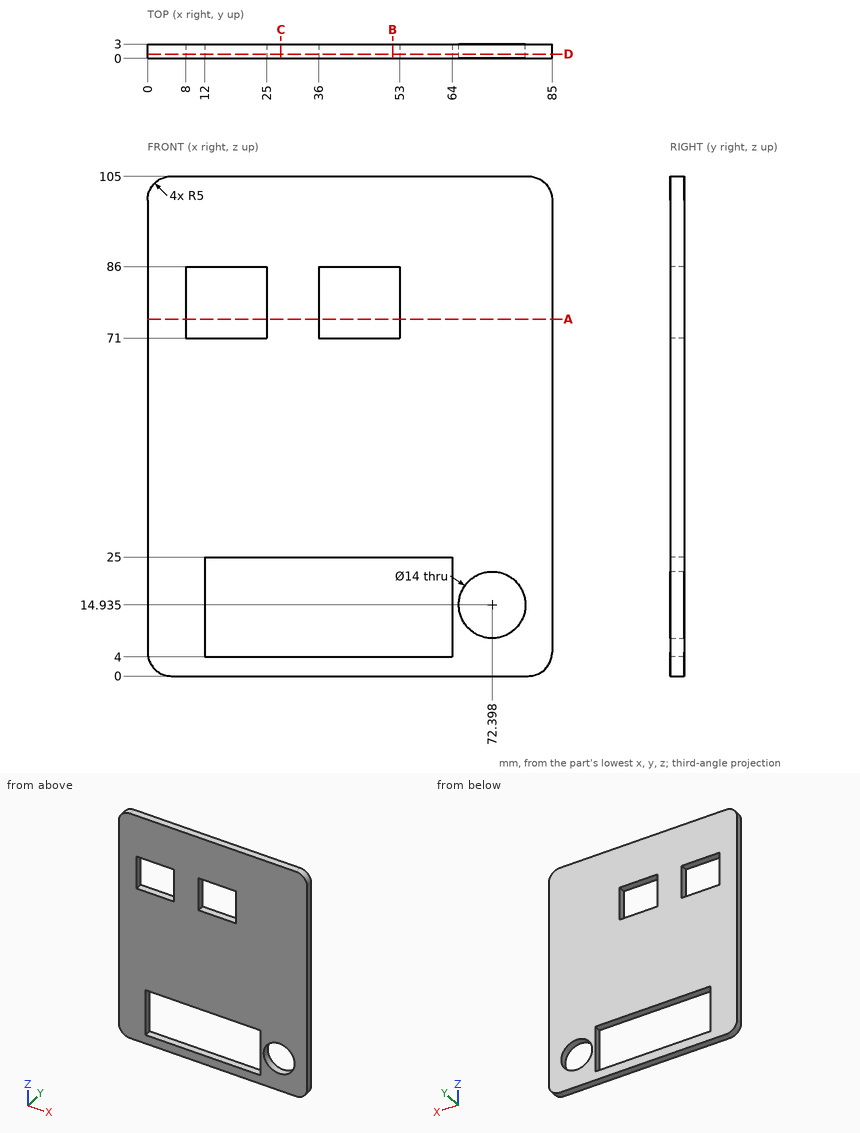
For this review, use the dimensioned drawing (mm, ordinates from the lowest corner) and the shaded views. Give positions to 0.01 mm unless a question says otherwise; leave off trailing zeros. Order: outer loops, then holes, each group sorted by start corner. A loop starts at its lowest first (then second) coordinate and runs counter-clockwise, first axis right, second up.
1) Take a section at A-A (z = 75). Give the boundary of the cut face in (x, y).
2) Take a section at B-B (x = 51.5). Give the boundary of the cut face in (y, z).
3) Wall thickness on line 1 (Z direction, x = 50.5, y = 1.4); line 2 (X direction, y = 2.05, z = 74.5); line 3 (Z direction, x = 54.5, y = 2.15): over which ranges is each line inside the solid? List them lowest first.
4) Take a section at C-C (x = 28). Give the boundary of the cut face in (y, z).
5) Take a section at D-D (y = 0.85). Give the boundary of the cut face in (x, z) (1 decimal), then the cut area to 3 significant figures.
Derived:
1. outline: (0, 0) - (8, 0) - (8, 3) - (0, 3) - close; (25, 0) - (36, 0) - (36, 3) - (25, 3) - close; (53, 0) - (85, 0) - (85, 3) - (53, 3) - close
2. outline: (0, 0) - (3, 0) - (3, 4) - (0, 4) - close; (0, 25) - (3, 25) - (3, 71) - (0, 71) - close; (0, 86) - (3, 86) - (3, 105) - (0, 105) - close
3. line 1: z = 0 to 4, 25 to 71, 86 to 105
3. line 2: x = 0 to 8, 25 to 36, 53 to 85
3. line 3: z = 0 to 4, 25 to 105
4. outline: (0, 0) - (3, 0) - (3, 4) - (0, 4) - close; (0, 25) - (3, 25) - (3, 105) - (0, 105) - close
5. outline: (0, 5) arc R5 ccw to (5, 0) - (80, 0) arc R5 ccw to (85, 5) - (85, 100) arc R5 ccw to (80, 105) - (5, 105) arc R5 ccw to (0, 100) - close; hole (8, 71) - (25, 71) - (25, 86) - (8, 86) - close; hole (12, 4) - (64, 4) - (64, 25) - (12, 25) - close; hole (36, 71) - (53, 71) - (53, 86) - (36, 86) - close; hole circle Ø14 at (72.4, 14.9)
5. area: 7,150 mm2
